Source: CAD feature listing. Evaluate the final solid. Frame: model axes, mm. A direction names the side the tool comes from. Round coordinates to 2 decimals unless told otherwise and drop trailing zeros. Order: outer loops, then holes, each group sorted by start corner. A loop starts at its lowest first (then second) coordinate and runs counter-clockwise, first axis right, second up. Notation, with made-up numbers: (-24, 5.5) - (-9, 5.5) arc R14 ccw to (-9, 27.5) - close; hole circle Ø11 at (19, -25.75). An arc over 180 degrees is marked (long way). Use one line per item in the form item = value. Start each with the question number.
Q1. Pin query (flat end, axial travel): pin 1 Ø0.8 at (y, z) = (3, 4) entering from -X; pin 2 Ø1.4 at (y, z) = (2.5, 4) entering from +X; pin 3 Ø4.5 at (x, y) = (30, 0) entering from +Z. Return the tip coordinate at first contact, or that it passes through.
Q2. Ray query, line 1 (Y direction, x = 30, z = 1.6); line 2 (Z direction, x = -16.5, y = -4). Return the intervals inside material, ascending. Write a range as [from, to].
Q3. Cut plane B-B, the plane z = 0.85. Return the cut outline in (x, y).
Q4. Set-up query: faces 5 (the flat face through (25, 3, 3)), 6 (the flat face through (15.31, 2.38, 3.63)), 7 (the flat face through (17.333, 3, 3)). Return all of +Z, -Z, +X, -X, +Y, -Y with unobstructed straight access to the full face (end or side cutting, diameter ignored); none if empty.
Q5. Draft query along X for faces 1 (the flat face through (22.97, 2.38, 3.63)), 2 (the cylindrical face through (29.19, 4.76, 4.23)), 3 (the cylindrical face through (-29.19, 4.76, 4.23)), 4 (the cylindrical face through (28.25, 0.08, 1.13)). Return one class per face: released by +X, released by -X, zero draft, split by the parting line, or undercut.
Q6. Cut plane A-A, the plane y = 0. Return the cut outline in (x, z), and give its area (3 significant figures).
from build123d import *

# Parameters (mm, degrees)
F0_R     = 1.75
F1_DEPTH = 2.3
F0_W     = 60
F0_H     = 2
F2_DEPTH = 5
F3_W     = 4
F3_H     = 2.7
F4_DEPTH = 2.7
F5_SIZE  = 2.69999
F6_R     = 2.69999


# Not quite as in the source:
# - a fillet or chamfer is up to 0.001 mm smaller than in the source, because OpenCascade refuses the exact size


with BuildPart() as f1:
    # F0 (on Top) → F1 (new body)
    with BuildSketch(Plane.XY):
        with BuildLine():
            Line((-30, 3.75), (-30, 5.75))
            ThreePointArc((-30, 5.75), (-35.75, 0), (-30, -5.75))
            Line((-30, -5.75), (30, -5.75))
            ThreePointArc((30, -5.75), (35.75, 0), (30, 5.75))
            Line((30, 5.75), (30, 3.75))
            Line((30, 3.75), (-30, 3.75))
        make_face()
        with Locations((-30, 0)):
            Circle(F0_R, mode=Mode.SUBTRACT)
        with Locations((30, 0)):
            Circle(F0_R, mode=Mode.SUBTRACT)
    extrude(amount=F1_DEPTH)

    # F0 (on Top) → F2 (join)
    with BuildSketch(Plane.XY):
        with Locations((0, 4.75)):
            Rectangle(F0_W, F0_H)
    extrude(amount=F2_DEPTH)

    # F3 (on face) → F4 (join, through all)
    with BuildSketch(Plane.XY.offset(2.3)):
        with Locations((-23, 2.4)):
            Rectangle(F3_W, F3_H)
        with Locations((-15.3333333333, 2.4)):
            Rectangle(F3_W, F3_H)
        with Locations((-7.6666666667, 2.4)):
            Rectangle(F3_W, F3_H)
        with Locations((0, 2.4)):
            Rectangle(F3_W, F3_H)
        with Locations((7.6666666667, 2.4)):
            Rectangle(F3_W, F3_H)
        with Locations((15.3333333333, 2.4)):
            Rectangle(F3_W, F3_H)
        with Locations((23, 2.4)):
            Rectangle(F3_W, F3_H)
    extrude(amount=F4_DEPTH)

    # F5 (size 2.7 in the source; OpenCascade refuses exactly that, so slightly less here)
    f5_edges = [f1.edges().sort_by_distance(p)[0] for p in [
        (-23, 1.05, 5),
        (-15.333333, 1.05, 5),
        (-7.666667, 1.05, 5),
        (0, 1.05, 5),
        (7.666667, 1.05, 5),
        (15.333333, 1.05, 5),
        (23, 1.05, 5),
    ]]
    chamfer(f5_edges, length=F5_SIZE)

    # F6 (radius 2.7 in the source; OpenCascade refuses exactly that, so slightly less here)
    f6_edges = [f1.edges().sort_by_distance(p)[0] for p in [
        (30, 4.75, 5),
        (-30, 4.75, 5),
    ]]
    fillet(f6_edges, radius=F6_R)


solid = f1.part
Completed:
q1.pin_1 = -25
q1.pin_2 = 25
q1.pin_3 = 2.3
q2.line_1 = [-5.75, -1.75], [1.75, 5.75]
q2.line_2 = [0, 2.3]
q3.outline = (-30, -5.75) - (30, -5.75) arc R5.75 ccw to (30, 5.75) - (-30, 5.75) arc R5.75 ccw to start; hole circle Ø3.5 at (-30, 0); hole circle Ø3.5 at (30, 0)
q4.face_5 = +Z, +X, -Y
q4.face_6 = +Z, +X, -X, -Y
q4.face_7 = +Z, -Y
q5.face_1 = zero draft
q5.face_2 = released by +X
q5.face_3 = released by -X
q5.face_4 = undercut
q6.outline = (-35.75, 0) - (-31.75, 0) - (-31.75, 2.3) - (-35.75, 2.3) - close; (-28.25, 0) - (28.25, 0) - (28.25, 2.3) - (-28.25, 2.3) - close; (31.75, 0) - (35.75, 0) - (35.75, 2.3) - (31.75, 2.3) - close
q6.area = 148 mm2
